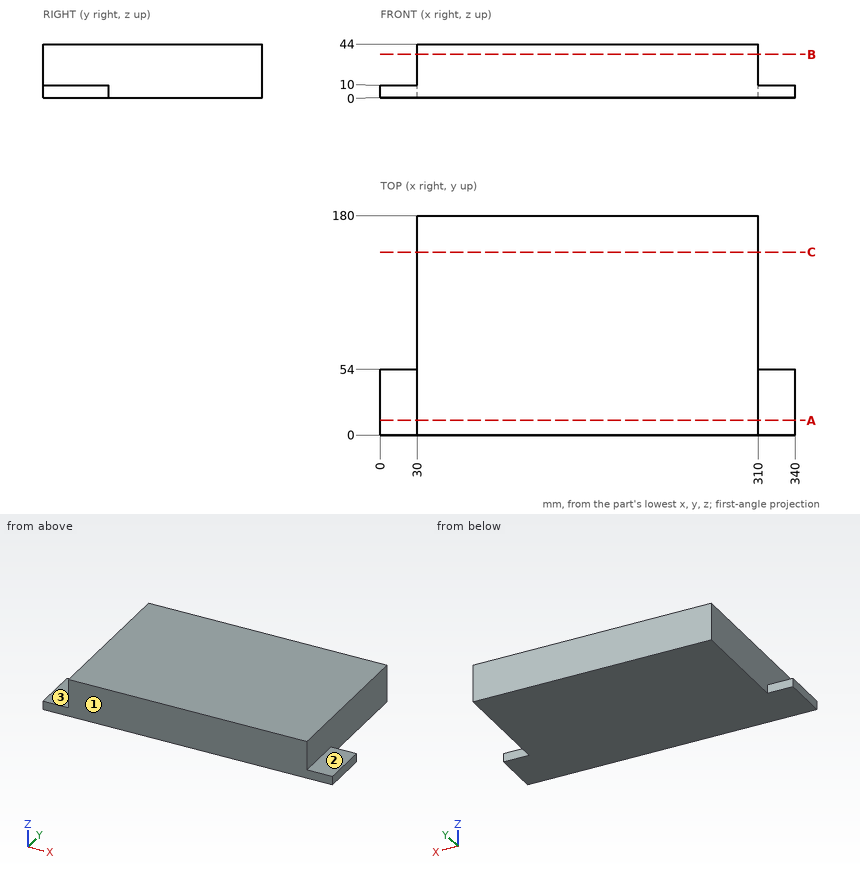
Could you check a few things on this drawing? It's one solid part, dimensions in mm from its lowest x, y, z. A direction names the side the tool comes from. Round coordinates to 2 decimals unless told otherwise and drop trailing zeros. Order: outer loops, then holes, each group sorted by start corner. A loop starts at its lowest first (then second) coordinate and runs counter-clockwise, first axis right, second up. Notation, with made-up numbers: (-30.75, 85.5) -> (-24.75, 85.5) arc R25 ccw to (-24.75, 122.5) -> close; hole circle Ø11 at (56, 52.25). An arc over 180 degrees is marked (long way). One line per question, with ' | ' between items.
Q1. Which directions (+Z, -Z, +X, -X, +Y, -Y) give clear straight access to the entire face, cutting with the end or side of a thin tool? Please do the marked faces 1, 2 and 3.
Computed values:
face 1: +Z, -Z, +X, -X, -Y | face 2: +Z, +X, +Y, -Y | face 3: +Z, -X, +Y, -Y
Q2. If we section it at C-C on y = 150: Write out the boundary of the cut face in (x, z).
Computed values:
outline: (30, 0) -> (310, 0) -> (310, 44) -> (30, 44) -> close
Q3. I'm going to push flat-ended pins straight in: pin 1 (6 mm diameter, centred on y = 59.5, z = 15, fed in from -X); pin 2 (8 mm diameter, centred on x = 320.5, z = 3, fed in from +Y); pin 3 (8 mm diameter, centred on x = 101, z = 20.5, fed in from -Y); pin 4 (22 mm diameter, centred on y = 48.5, z = 32.5, fed in from +X). Where does each tip first touch, or does it pass through?
Computed values:
pin 1: x = 30 | pin 2: y = 54 | pin 3: y = 0 | pin 4: x = 310
Q4. If we section it at B-B on z = 35.5: Write out the boundary of the cut face in (x, y), plus the area to 3 significant figures.
Computed values:
outline: (30, 0) -> (310, 0) -> (310, 180) -> (30, 180) -> close | area: 50,400 mm²
Q5. If we section it at A-A on y = 12: Write out the boundary of the cut face in (x, z), plus the area to 3 significant figures.
Computed values:
outline: (0, 0) -> (340, 0) -> (340, 10) -> (310, 10) -> (310, 44) -> (30, 44) -> (30, 10) -> (0, 10) -> close | area: 12,900 mm²
Q6. If I drill on line 1 (X direction, y = 133.5, z = 30.5), over which ranges is the centre line in solid material (lowest first)? Write a range as from..to.
Computed values:
line 1: 30..310
